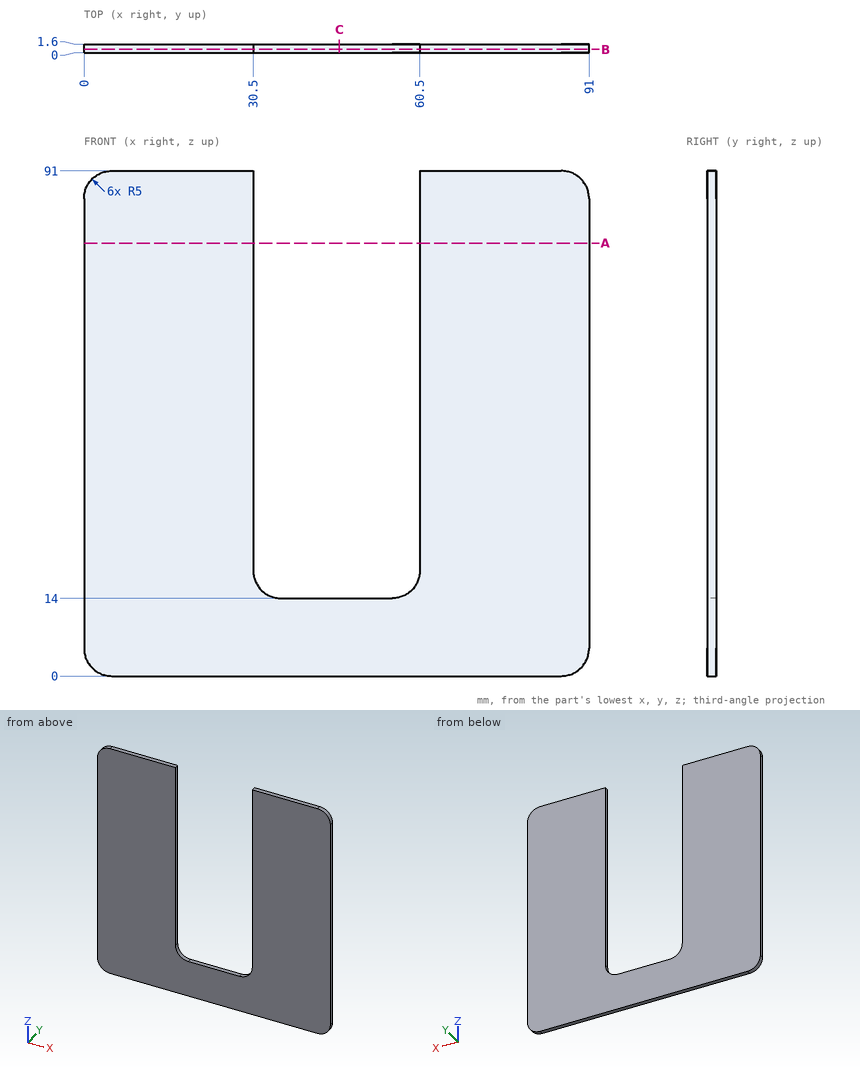
The drawing under review shows one solid part. Ordinate dimensions are in mm from its lowest x, y, z. Coordinates: 2 decimals unless noted, no trailing zeros. Loops run counter-clockwise (first coordinate to the right, second up) from the corner with the lowest first, then second, coordinate; pieces in that order, holes last.
Item 1: Add section B-B (y = 0.65). Write out the cut boundary in (x, z).
Completed:
outline: (0, 5) arc R5 ccw to (5, 0) - (86, 0) arc R5 ccw to (91, 5) - (91, 86) arc R5 ccw to (86, 91) - (60.5, 91) - (60.5, 19) arc R5 cw to (55.5, 14) - (35.5, 14) arc R5 cw to (30.5, 19) - (30.5, 91) - (5, 91) arc R5 ccw to (0, 86) - close
Item 2: Add section C-C (x = 46). Write out the cut boundary in (y, z).
Completed:
outline: (0, 0) - (1.6, 0) - (1.6, 14) - (0, 14) - close
Item 3: Add section A-A (z = 78). Write out the cut boundary in (x, y).
Completed:
outline: (0, 0) - (30.5, 0) - (30.5, 1.6) - (0, 1.6) - close; (60.5, 0) - (91, 0) - (91, 1.6) - (60.5, 1.6) - close
Item 4: Wall thickness on L1, parallel to X at y = 1.35, z = 33; L2, parallel to Z at x = 37.5, y = 0.35; L3, parallel to Z at x = 33, y = 1.1: over which ranges is each line inside the solid? List them lowest first.
Completed:
L1: x = 0 to 30.5, 60.5 to 91
L2: z = 0 to 14
L3: z = 0 to 14.67
Item 5: Clearance check with a flat-ended pin moving along its axis: pin 1 (4 mm diameter, centred on x = 30.5, z = 75.5, fed in from -Y). State where the tip first meets the part, or that it passes through.
Completed:
pin 1: stops at y = 0
